```python
from build123d import *

# Parameters (mm, degrees)
SKETCH1_R           = 3.5
SKETCH1_R_2         = 2.5
SKETCH1_R_3         = 2
BOSS_EXTRUDE2_DEPTH = 5


with BuildPart() as part:
    # Sketch1 → Boss-Extrude2 (new body)
    with BuildSketch(Plane(origin=(0, 0, 0), x_dir=(1, 0, 0), z_dir=(0, 1, 0))):
        with BuildLine():
            Line((-131.94689332, 25.970681882), (-134.592588801, 23.324986401))
            ThreePointArc((-134.592588801, 23.324986401), (-137.58868474, 17.60266792), (-139.140311552, 11.332582281))
            Line((-139.140311552, 11.332582281), (-139.140311552, -11.332582281))
            ThreePointArc((-139.140311552, -11.332582281), (-137.58868474, -17.60266792), (-134.592588801, -23.324986401))
            Line((-134.592588801, -23.324986401), (-131.94689332, -25.970681882))
            ThreePointArc((-131.94689332, -25.970681882), (-126.689188545, -30.877876968), (-122.964643548, -37.030257619))
            Line((-122.964643548, -37.030257619), (-113.128962492, -51.346084613))
            add(Edge.make_bspline(
                [(-84.396160179, -89.98721953), (-74.548053374, -70.617720847), (-84.125654145, -57.737342542), (-113.128962492, -51.346084613)],
                knots=[0.072527255, 0.072527255, 0.072527255, 0.072527255, 1, 1, 1, 1], degree=3))
            Line((-84.396160179, -89.98721953), (-80.477300699, -101.896066655))
            Line((-80.477300699, -101.896066655), (-74.796293078, -102.076946621))
            ThreePointArc((-74.796293078, -102.076946621), (-67.604609488, -99.92775096), (-62.778823596, -94.178738404))
            Line((-62.778823596, -94.178738404), (-52.387218797, -77.500760005))
            ThreePointArc((-52.387218797, -77.500760005), (-35.405083828, -65.014987094), (-18.42294886, -77.500760005))
            Line((-18.42294886, -77.500760005), (-7.983045495, -100.927738965))
            ThreePointArc((-7.983045495, -100.927738965), (-5.375974323, -105.279578897), (-0.95323828, -107.764480662))
            Line((-0.95323828, -107.764480662), (154.12105013, -107.764480662))
            ThreePointArc((154.12105013, -107.764480662), (157.84777942, -105.444091096), (160.179787775, -101.724621245))
            Line((160.179787775, -101.724621245), (176.051157754, -71.206455594))
            ThreePointArc((176.051157754, -71.206455594), (177.340217514, -68.190997819), (177.557153354, -64.918750962))
            Line((177.557153354, -64.918750962), (177.557153354, 64.918750962))
            ThreePointArc((177.557153354, 64.918750962), (177.340217514, 68.190997819), (176.051157754, 71.206455594))
            Line((176.051157754, 71.206455594), (160.179787775, 101.724621245))
            ThreePointArc((160.179787775, 101.724621245), (157.84777942, 105.444091096), (154.12105013, 107.764480662))
            Line((154.12105013, 107.764480662), (-0.95323828, 107.764480662))
            ThreePointArc((-0.95323828, 107.764480662), (-5.375974323, 105.279578897), (-7.983045495, 100.927738965))
            Line((-7.983045495, 100.927738965), (-18.42294886, 77.500760005))
            ThreePointArc((-18.42294886, 77.500760005), (-35.405083828, 65.014987094), (-52.387218797, 77.500760005))
            Line((-52.387218797, 77.500760005), (-62.778823596, 94.178738404))
            ThreePointArc((-62.778823596, 94.178738404), (-67.604609488, 99.92775096), (-74.796293078, 102.076946621))
            Line((-74.796293078, 102.076946621), (-80.477300699, 101.896066655))
            Line((-80.477300699, 101.896066655), (-84.396160179, 89.98721953))
            add(Edge.make_bspline(
                [(-84.396160179, 89.98721953), (-74.548053374, 70.617720847), (-84.125654145, 57.737342542), (-113.128962492, 51.346084613)],
                knots=[0.072527255, 0.072527255, 0.072527255, 0.072527255, 1, 1, 1, 1], degree=3))
            Line((-113.128962492, 51.346084613), (-122.964643548, 37.030257619))
            ThreePointArc((-122.964643548, 37.030257619), (-126.689188545, 30.877876968), (-131.94689332, 25.970681882))
        make_face()
        with Locations((145.5, 70.5)):
            Circle(SKETCH1_R, mode=Mode.SUBTRACT)
        with Locations((4.5, 70.5)):
            Circle(SKETCH1_R, mode=Mode.SUBTRACT)
        with Locations((4.5, -70.5)):
            Circle(SKETCH1_R, mode=Mode.SUBTRACT)
        with Locations((145.5, -70.5)):
            Circle(SKETCH1_R, mode=Mode.SUBTRACT)
        with Locations((-73.905296724, 97.603035068)):
            Circle(SKETCH1_R_2, mode=Mode.SUBTRACT)
        with Locations((-36.642164959, 36.630202961)):
            Circle(SKETCH1_R_2, mode=Mode.SUBTRACT)
        with Locations((-36.642164959, -36.630202961)):
            Circle(SKETCH1_R_2, mode=Mode.SUBTRACT)
        with Locations((-73.905296724, -97.603035068)):
            Circle(SKETCH1_R_2, mode=Mode.SUBTRACT)
        with Locations((-109.755224174, -27.254093608)):
            Circle(SKETCH1_R_2, mode=Mode.SUBTRACT)
        with Locations((-109.755224174, -41.994093608)):
            Circle(SKETCH1_R_2, mode=Mode.SUBTRACT)
        with Locations((-109.755224174, 41.994093608)):
            Circle(SKETCH1_R_2, mode=Mode.SUBTRACT)
        with Locations((-109.755224174, 27.254093608)):
            Circle(SKETCH1_R_2, mode=Mode.SUBTRACT)
        with Locations((133.617169417, -84.482617886)):
            Circle(SKETCH1_R_3, mode=Mode.SUBTRACT)
        with Locations((133.617169417, 84.482617886)):
            Circle(SKETCH1_R_3, mode=Mode.SUBTRACT)
        with Locations((133.617169417, 98.534958019)):
            Circle(SKETCH1_R_3, mode=Mode.SUBTRACT)
        with BuildLine():
            Line((22.641562111, -35.632069218), (22.641562111, 36.652844088))
            ThreePointArc((22.641562111, 36.652844088), (20.608136604, 40.692979265), (16.151822888, 41.466787774))
            ThreePointArc((16.151822888, 41.466787774), (5.788194255, 40.650697554), (-3.683793295, 36.366744527))
            Line((-3.683793295, 36.366744527), (-14.203195163, 28.148087048))
            ThreePointArc((-14.203195163, 28.148087048), (-16.255277744, 26.678740586), (-18.42294886, 25.385982343))
            ThreePointArc((-18.42294886, 25.385982343), (-21.506931984, 22.427406429), (-22.641562111, 18.307122723))
            Line((-22.641562111, 18.307122723), (-22.641562111, -17.286347854))
            ThreePointArc((-22.641562111, -17.286347854), (-21.506931984, -21.40663156), (-18.42294886, -24.365207473))
            ThreePointArc((-18.42294886, -24.365207473), (-16.255277744, -25.657965716), (-14.203195163, -27.127312178))
            Line((-14.203195163, -27.127312178), (-3.683793295, -35.345969657))
            ThreePointArc((-3.683793295, -35.345969657), (5.788194255, -39.629922684), (16.151822888, -40.446012904))
            ThreePointArc((16.151822888, -40.446012904), (16.873563182, -40.607991845), (17.611254517, -40.662376812))
            ThreePointArc((17.611254517, -40.662376812), (21.168219128, -39.189033829), (22.641562111, -35.632069218))
        make_face(mode=Mode.SUBTRACT)
        with BuildLine():
            Line((-89.554671241, 41.117352002), (-99.147214694, 20.593394094))
            ThreePointArc((-99.147214694, 20.593394094), (-99.888375125, 19.267909053), (-100.81360523, 18.063675425))
            add(Edge.make_bspline(
                [(-100.81360523, 18.063675425), (-110.428458968, 7.271163587), (-110.428458968, -7.271012097), (-100.81360523, -18.063523935)],
                knots=[3.977868885, 3.977868885, 3.977868885, 3.977868885, 5.446909075, 5.446909075, 5.446909075, 5.446909075], degree=3, weights=[1, 0.828101657, 0.828101657, 1]))
            ThreePointArc((-100.81360523, -18.063523935), (-99.888375125, -19.267757563), (-99.147214694, -20.593242605))
            Line((-99.147214694, -20.593242605), (-89.554671241, -41.117200512))
            ThreePointArc((-89.554671241, -41.117200512), (-85.693735649, -45.513878761), (-80.075843646, -47.15))
            Line((-80.075843646, -47.15), (-78.905296724, -47.15))
            ThreePointArc((-78.905296724, -47.15), (-74.062527173, -45.961807095), (-70.319656797, -42.667093047))
            Line((-70.319656797, -42.667093047), (-59.297241663, -26.842279456))
            ThreePointArc((-59.297241663, -26.842279456), (-54.702966705, -23.150586853), (-48.842250779, -22.527718094))
            ThreePointArc((-48.842250779, -22.527718094), (-48.370274947, -22.61640832), (-47.899419977, -22.710868575))
            Line((-47.899419977, -22.710868575), (-46.142268668, -23.074578438))
            ThreePointArc((-46.142268668, -23.074578438), (-45.878558587, -23.115265356), (-45.612075542, -23.128874868))
            ThreePointArc((-45.612075542, -23.128874868), (-43.762453944, -22.362736517), (-42.996315593, -20.51311492))
            Line((-42.996315593, -20.51311492), (-42.996315593, 20.513266409))
            ThreePointArc((-42.996315593, 20.513266409), (-43.762453944, 22.362888007), (-45.612075542, 23.129026358))
            ThreePointArc((-45.612075542, 23.129026358), (-45.878558587, 23.115416846), (-46.142268668, 23.074729928))
            Line((-46.142268668, 23.074729928), (-47.899419977, 22.711020065))
            ThreePointArc((-47.899419977, 22.711020065), (-48.370274947, 22.61655981), (-48.842250779, 22.527869583))
            ThreePointArc((-48.842250779, 22.527869583), (-49.773143794, 22.401695376), (-50.711601736, 22.359523992))
            ThreePointArc((-50.711601736, 22.359523992), (-55.554371288, 23.547716898), (-59.297241663, 26.842430946))
            Line((-59.297241663, 26.842430946), (-71.047432728, 43.712107962))
            ThreePointArc((-71.047432728, 43.712107962), (-75.193394119, 46.552119459), (-80.183151299, 47.149601208))
            ThreePointArc((-80.183151299, 47.149601208), (-85.738926275, 45.485105607), (-89.554671241, 41.117352002))
        make_face(mode=Mode.SUBTRACT)
        with BuildLine():
            Line((144.587268898, 54.298841595), (144.587268898, 54.751074521))
            ThreePointArc((144.587268898, 54.751074521), (141.136808174, 64.355010875), (132.363285671, 69.567167393))
            ThreePointArc((132.363285671, 69.567167393), (128.85387667, 71.65203), (127.47369238, 75.493604542))
            Line((127.47369238, 75.493604542), (127.47369238, 83.46456071))
            ThreePointArc((127.47369238, 83.46456071), (123.732967698, 93.409858769), (114.365288749, 98.424693337))
            ThreePointArc((114.365288749, 98.424693337), (111.397974334, 98.718864685), (108.417731298, 98.8170638))
            Line((108.417731298, 98.8170638), (90.123559862, 98.8170638))
            ThreePointArc((90.123559862, 98.8170638), (81.586844795, 95.281040642), (78.050821636, 86.744325575))
            Line((78.050821636, 86.744325575), (78.050821636, 54.298841595))
            ThreePointArc((78.050821636, 54.298841595), (79.818833216, 50.030484062), (84.087190749, 48.262472483))
            Line((84.087190749, 48.262472483), (138.550899786, 48.262472483))
            ThreePointArc((138.550899786, 48.262472483), (142.819257319, 50.030484062), (144.587268898, 54.298841595))
        make_face(mode=Mode.SUBTRACT)
        with BuildLine():
            Line((84.087190749, -48.262472483), (138.550899786, -48.262472483))
            ThreePointArc((138.550899786, -48.262472483), (142.819257319, -50.030484062), (144.587268898, -54.298841595))
            Line((144.587268898, -54.298841595), (144.587268898, -54.751074521))
            ThreePointArc((144.587268898, -54.751074521), (141.136808174, -64.355010875), (132.363285671, -69.567167393))
            ThreePointArc((132.363285671, -69.567167393), (128.85387667, -71.65203), (127.47369238, -75.493604542))
            Line((127.47369238, -75.493604542), (127.47369238, -83.46456071))
            ThreePointArc((127.47369238, -83.46456071), (123.732967698, -93.409858769), (114.365288749, -98.424693337))
            ThreePointArc((114.365288749, -98.424693337), (111.397974334, -98.718864685), (108.417731298, -98.8170638))
            Line((108.417731298, -98.8170638), (90.123559862, -98.8170638))
            ThreePointArc((90.123559862, -98.8170638), (81.586844795, -95.281040642), (78.050821636, -86.744325575))
            Line((78.050821636, -86.744325575), (78.050821636, -54.298841595))
            ThreePointArc((78.050821636, -54.298841595), (79.818833216, -50.030484062), (84.087190749, -48.262472483))
        make_face(mode=Mode.SUBTRACT)
        with BuildLine():
            ThreePointArc((31.641562111, 4.798271927), (33.641562111, 6.798271927), (31.641562111, 8.798271927))
            ThreePointArc((31.641562111, 8.798271927), (29.641562111, 6.798271927), (31.641562111, 4.798271927))
        make_face(mode=Mode.SUBTRACT)
        with BuildLine():
            ThreePointArc((31.641562111, -7.681612107), (33.641562111, -5.681612107), (31.641562111, -3.681612107))
            ThreePointArc((31.641562111, -3.681612107), (29.641562111, -5.681612107), (31.641562111, -7.681612107))
        make_face(mode=Mode.SUBTRACT)
        with BuildLine():
            ThreePointArc((109.877976865, 4.478055975), (105.350700031, -0.04922086), (109.877976865, -4.576497694))
            ThreePointArc((109.877976865, -4.576497694), (114.4052537, -0.04922086), (109.877976865, 4.478055975))
        make_face(mode=Mode.SUBTRACT)
        with BuildLine():
            ThreePointArc((-31.641562111, -3.681612107), (-29.641562111, -5.681612107), (-31.641562111, -7.681612107))
            ThreePointArc((-31.641562111, -7.681612107), (-33.641562111, -5.681612107), (-31.641562111, -3.681612107))
        make_face(mode=Mode.SUBTRACT)
        with BuildLine():
            ThreePointArc((-31.641562111, 8.798271927), (-29.641562111, 6.798271927), (-31.641562111, 4.798271927))
            ThreePointArc((-31.641562111, 4.798271927), (-33.641562111, 6.798271927), (-31.641562111, 8.798271927))
        make_face(mode=Mode.SUBTRACT)
    extrude(amount=BOSS_EXTRUDE2_DEPTH)


solid = part.part
```
Here's how the part is built. I have some questions about the finished solid (model axes, mm). A direction names the side the tool comes from. Round coordinates to 2 decimals unless told otherwise and drop trailing zeros. Loops run counter-clockwise (first coordinate to the right, second up) from the corner with the lowest first, then second, coordinate; pieces in that order, holes last.
1. If I drill on probe 1 along X at (y, z) = (3.55, 6); probe 2 along X at (y, z) = (4.6, 70.5); probe 3 along Z at (x, y) = (4.5, 1.6), over which ranges is the centre line in solid material (lowest first)?
Answers:
probe 1: x = -139.14 to -107, -43 to -33.62, -29.67 to -22.64, 22.64 to 29.67, 33.62 to 177.56
probe 2: x = -81.66 to -48.25, -22.56 to 1, 8 to 78.05, 130.12 to 142, 149 to 176.47
probe 3: z = -107.76 to -74, -67 to -40.29, 39.27 to 67, 74 to 107.76
2. Thinking about a two-plate mould opening in X: for faces 6 (the face through (-126.753, 2.465, 30.8)), 7 (the face through (168.004, 2.465, 86.679)), 8 (the face through (123.83, 2.46, 93.3)), which applies, released by +X, released by -X, zero draft, split by the parting line, or undercut?
Answers:
face 6: released by -X
face 7: released by +X
face 8: undercut
3. Will these pins go through, and if not, where does the flat tip stop? pin 1 (4.5 mm diameter, centred on x = -109.76, z = -41.99, fed in from +Y); pin 2 (1.5 mm diameter, centred on y = 3, z = -67, fed in from -X); pin 3 (1 mm diameter, centred on y = 1.5, z = -49, fed in from +X).
Answers:
pin 1: passes through
pin 2: stops at x = -83.87
pin 3: stops at x = 177.56
4. Suppose I cut it at B-B, the plane y = 1.05. Give the number of separate pieces and of enclosed holes in the cut face, and give its area (3 significant figures).
Answers:
separate pieces: 1
enclosed holes: 24
area: 43,400 mm2
5. For faces 1 (the face through (168.2, 2.5, -86.3)), 2 (the face through (-57.66, 2.46, 85.96)), 3 (the face through (-13.13, 2.46, -89.38)), 4 (the face through (-9.017, 2.465, 31.179)), 5 (the face through (157.8, 2.46, 105.49)), which set-ups out of +Z, -Z, +X, -X, +Y, -Y let a thin tool reach every point of the face, with its end or its side?
Answers:
face 1: -Z, +X, +Y, -Y
face 2: +Z, +Y, -Y
face 3: -Z, +Y, -Y
face 4: +Y, -Y
face 5: +Z, +X, +Y, -Y
6. Suppose I cut it at A-A, the plane x = 4.5. Please give me the cut outline in (y, z), and give its area (3 significant figures).
Answers:
outline: (0, -107.76) - (5, -107.76) - (5, -74) - (0, -74) - close; (0, -67) - (5, -67) - (5, -40.29) - (0, -40.29) - close; (0, 39.27) - (5, 39.27) - (5, 67) - (0, 67) - close; (0, 74) - (5, 74) - (5, 107.76) - (0, 107.76) - close
area: 610 mm2
